Autodesk Inventor part; units mm, degrees
ref_plane "YZ Plane" through (0, 0, 0) normal (1, 0, 0) x (0, 1, 0)
ref_plane "XZ Plane" through (0, 0, 0) normal (0, 1, 0) x (-1, 0, 0)
ref_plane "XY Plane" through (0, 0, 0) normal (0, 0, 1) x (1, 0, 0)
sketch "スケッチ1" plane through (0, 0, 0) normal (0, 1, 0) x (-1, 0, 0)
  line L0 (0, 0) -> (0, -24) construction
  circle A0 centre (0, -24) radius 5
  arc A1 (-9.3528, -20.4608) -> (9.3528, -20.4608) centre (0, -24) ccw
  line L1 (11, -2) -> (-11, -2) construction
  line L2 (-11, -2) -> (-11, 2)
  line L3 (11, 2) -> (11, -2)
  line L4 (11, 0) -> (-11, 0) construction
  circle A2 centre (8, 0) radius 1.05
  circle A3 centre (-8, 0) radius 1.05
  circle A4 centre (0, -24) radius 8 construction
  circle A5 centre (5.6569, -18.3431) radius 1.05
  circle A6 centre (0, -16) radius 1.05
  circle A7 centre (-5.6569, -18.3431) radius 1.05
  circle A8 centre (-8, -24) radius 1.05
  circle A9 centre (-5.6569, -29.6569) radius 1.05
  circle A10 centre (0, -32) radius 1.05
  circle A11 centre (5.6569, -29.6569) radius 1.05
  circle A12 centre (8, -24) radius 1.05
  line L5 (-3.05, 2) -> (-3.05, -0.9893)
  line L6 (-3.05, -2.05) -> (-1.9893, -2.05) construction
  arc A13 (1.9893, -2.05) -> (3.05, -0.9893) centre (2.5197, -1.5197) ccw
  line L7 (3.05, -2.05) -> (2.5197, -1.5197) construction
  line L8 (3.05, -0.9893) -> (3.05, 2)
  arc A14 (-3.05, -0.9893) -> (-1.9893, -2.05) centre (-2.5197, -1.5197) ccw
  line L9 (-3.05, -2.05) -> (-2.5197, -1.5197) construction
  line L10 (-3.05, -0.9893) -> (-3.05, -2.05) construction
  line L11 (-1.9893, -2.05) -> (1.9893, -2.05)
  line L12 (3.05, -0.9893) -> (3.05, -2.05) construction
  line L13 (1.9893, -2.05) -> (3.05, -2.05) construction
  line L14 (-11, 2) -> (-3.05, 2)
  line L15 (3.05, 2) -> (11, 2)
  arc A15 (10.863, -2.5052) -> (11, -2) centre (10, -2) ccw
  arc A16 (10.863, -2.5052) -> (9.3528, -20.4608) centre (28.9008, -13.0637) ccw
  line L16 (8, -6.3971) -> (8, -16.9723) construction
  arc A17 (-11, -2) -> (-10.863, -2.5052) centre (-10, -2) ccw
  arc A18 (-9.3528, -20.4608) -> (-10.863, -2.5052) centre (-28.9008, -13.0637) ccw
  dimension "d18" = 16
  dimension "d0" = 22
  dimension "d1" = 10
  dimension "d2" = 10
  dimension "d5" = 16
  dimension "d6" = 2.1
  dimension "d16" = 360
  dimension "d19" = 2.1
  dimension "d20" = 22
  dimension "d23" = 0.75
  dimension "d26" = 6.1
  dimension "d28" = 45
  dimension "d29" = 0.75
  dimension "d30" = 45
  dimension "d32" = 4
  dimension "d33" = 4.05
  dimension "d34" = 1
  dimension "d35" = 16
extrude "押し出し1" add sketch "スケッチ1" along normal blind 2
chamfer "面取り1" distance 0.25 angle 45 4 edges at (11, 1, 2) (-11, 1, 2) (-3.05, 1, 2) (3.05, 1, 2)
properties part number "16_008_COXA_FRAME_3_R1" material "Aluminum 6061"
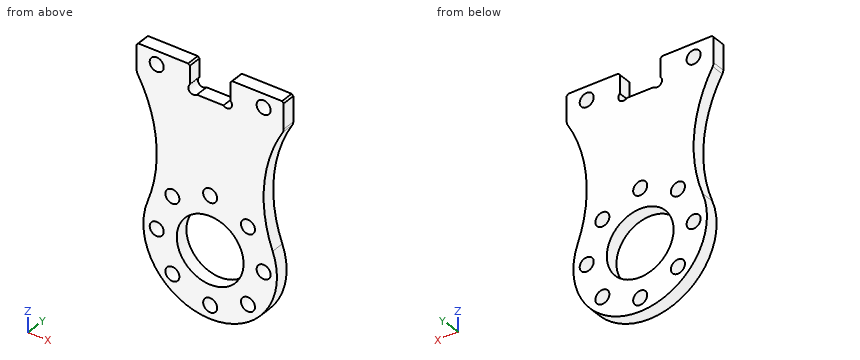
Geometry check sheet. Reference: the model listing, model coordinates, mm. Coordinates: 2 decimals unless noted, no trailing zeros. Order: outer loops, then holes, each group sorted by start corner. A loop starts at its lowest first (then second) coordinate and runs counter-clockwise, first axis right, second up.
Q1. Sectioned sample at A-A on x = 0. Record the cut outline in (y, z), and give its area (3 significant figures).
Reply:
outline: (0, -34) - (2, -34) - (2, -33.05) - (0, -33.05) - close; (0, -30.95) - (2, -30.95) - (2, -29) - (0, -29) - close; (0, -19) - (2, -19) - (2, -17.05) - (0, -17.05) - close; (0, -14.95) - (2, -14.95) - (2, -2.05) - (0, -2.05) - close
area: 35.5 mm2
Q2. Thickness scan on probe 1 along Z at (x, y) = (0, 1.15); probe 2 along Z at (x, y) = (5.5, 0.75); probe 3 along Z at (x, y) = (-7.25, 0.5). Record the ranges inside material, lowest first.
Reply:
probe 1: z = -34 to -33.05, -30.95 to -29, -19 to -17.05, -14.95 to -2.05
probe 2: z = -32.35 to -30.7, -28.62 to -19.38, -17.3 to 2
probe 3: z = -30.89 to -24.73, -23.27 to -0.73, 0.73 to 2
Q3. Sectioned sample at B-B on y = 1.15. Give the number of separate pieces and of enclosed holes in the cut face, and give its area (3 significant figures).
Reply:
separate pieces: 1
enclosed holes: 11
area: 500 mm2
Q4. Sectioned sample at C-C on x = 2.5. Record the cut outline in (y, z).
Reply:
outline: (0, -33.68) - (2, -33.68) - (2, -28.33) - (0, -28.33) - close; (0, -19.67) - (2, -19.67) - (2, -2.27) - (0, -2.27) - close
Q5. Depth check by flat-ended pin: pin 1 Ø1.7 at (x, z) = (5.66, -29.66) entering from +Y; pin 2 Ø0.6 at (x, y) = (0, 0.5) entering from +Z. Enter the tip coordinate at first touch or a pass-through.
Reply:
pin 1: passes through
pin 2: stops at z = -2.05
Q6. Sectioned sample at D-D on z = -16. Record the cut outline in (x, y), and give its area (3 significant figures).
Reply:
outline: (-8.21, 0) - (-1.05, 0) - (-1.05, 2) - (-8.21, 2) - close; (1.05, 0) - (8.21, 0) - (8.21, 2) - (1.05, 2) - close
area: 28.6 mm2
